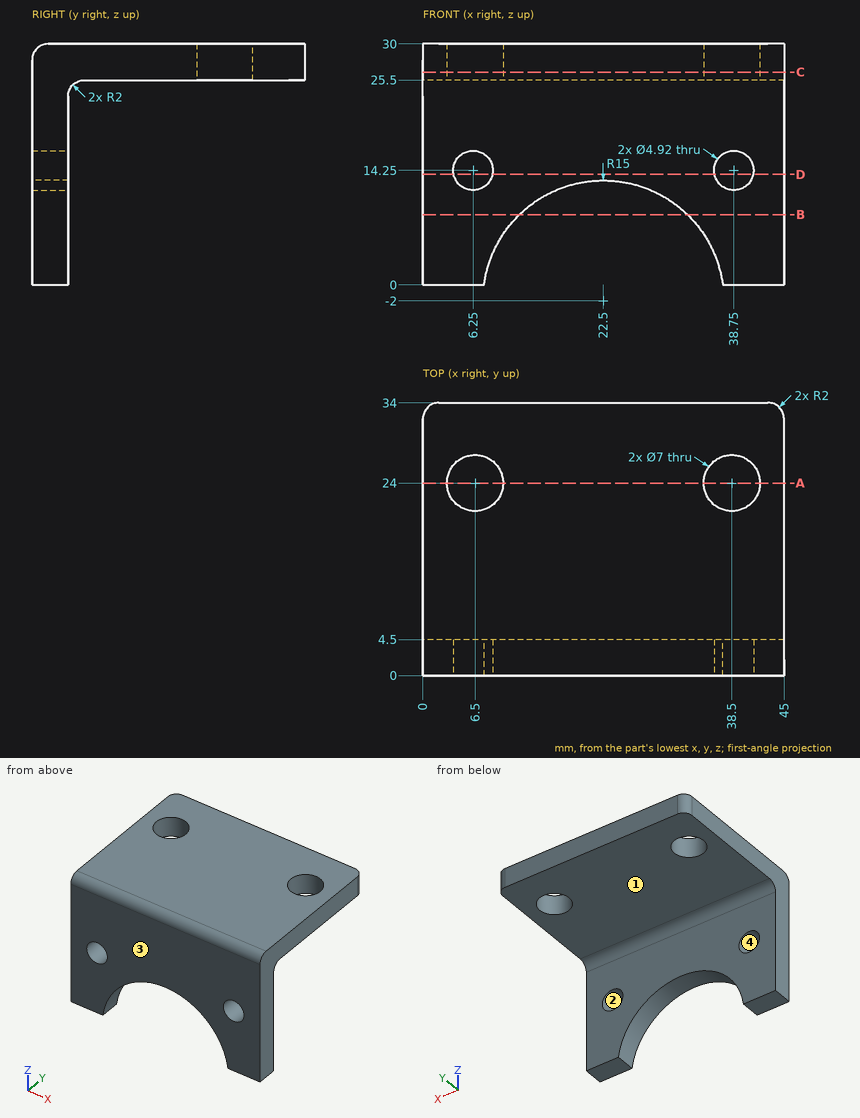
Design review of the part shown in the three views and the two pictorial views. Dimensions are in mm from the part's minimum x, y and z. A direction names the side the tool comes from. Round coordinates to 2 decimals unless told otherwise and drop trailing zeros. Order: outer loops, then holes, each group sorted by start corner. A loop starts at its lowest first (then second) coordinate and runs counter-clockwise, first axis right, second up. Notation, with made-up numbers: M -5,-31.75 L 29,-31.75 A23 ccw 29,-11.75 Z; hole C 79,29.5 d9. An arc over 180 degrees is marked long. Put each result on its own line as item: value.
Q1. Machinability: for the marked faces 1 and 2, which of the approach directions +Z, -Z, +X, -X, +Y, -Y give a long, thin tool a straight path to every point of the face, cutting with its end or side? Answer none if there is none.
Reported:
face 1: -Z, +X, -X, +Y
face 2: +Y, -Y
Q2. Consider section A-A (y = 24). State the section outline as (x, z) points, and give its area (4 significant figures).
Reported:
outline: M 0,25.5 L 3,25.5 L 3,30 L 0,30 Z; M 10,25.5 L 35,25.5 L 35,30 L 10,30 Z; M 42,25.5 L 45,25.5 L 45,30 L 42,30 Z
area: 139.5 mm²
Q3. Insertion check: pin 1 Ø3 at (x, y) = (38, 20.5) entering from -Z; pin 2 Ø2 at (x, y) = (35, 5) entering from -Z; pin 3 Ø11 at (x, y) = (6.5, 24) entering from +Z; pin 4 Ø6.5 at (x, z) = (38.75, 14.25) entering from +Y. Each pin has a flat end and moves straight along its axis. Give the tip position at first contact, or say it passes through.
Reported:
pin 1: z = 25.5
pin 2: z = 4.81
pin 3: z = 30
pin 4: y = 4.5
Q4. Consider section B-B (z = 8.75). State the section outline as (x, y) points.
Reported:
outline: M 0,0 L 12.04,0 L 12.04,4.5 L 0,4.5 Z; M 32.96,0 L 45,0 L 45,4.5 L 32.96,4.5 Z
Q5. Consider section C-C (z = 26.5). State the section outline as (x, y) points, and give its area (3 significant figures).
Reported:
outline: M 0,0 L 45,0 L 45,32 A2 ccw 43,34 L 2,34 A2 ccw 0,32 Z; hole C 6.5,24 d7; hole C 38.5,24 d7
area: 1,450 mm²
Q6. Draft analysis for pull direction X (two halves, no side actions). For the marked faces 3 and 4, state which applies: released by +X, released by -X, zero draft, split by the parting line, or undercut.
Reported:
face 3: zero draft
face 4: undercut
Q7. Consider section D-D (z = 13.75). State the section outline as (x, y) points, and give its area (3 significant figures).
Reported:
outline: M 0,0 L 3.84,0 L 3.84,4.5 L 0,4.5 Z; M 8.66,0 L 36.34,0 L 36.34,4.5 L 8.66,4.5 Z; M 41.16,0 L 45,0 L 45,4.5 L 41.16,4.5 Z
area: 159 mm²
Q8. To check wall thickness, follow line 1 (X direction, y = 3.1, z = 14.25); line 2 (X direction, y = 24, z = 28.1); line 3 (Z direction, x = 15.5, y = 29.5). State the ranges of each line that lie inside material, in increasing order.
Reported:
line 1: 0 to 3.79, 8.71 to 36.29, 41.21 to 45
line 2: 0 to 3, 10 to 35, 42 to 45
line 3: 25.5 to 30
